Source: CAD feature listing. Evaluate the final solid. Frame: model axes, mm. Give positions to 0.01 mm unless a question says otherwise; leave off trailing zeros. Order: outer loops, then holes, each group sorted by start corner. A loop starts at its lowest first (then second) coordinate and runs counter-clockwise, first axis right, second up. Notation, with made-up numbers: M 16,-20 L 25,-20 A15 cw 25,-12 Z; hole C 55,68.25 d8. An arc over 180 degrees is marked long. Use CSV: the item, a comma, the result in double quotes. Start each with the question number.
1. Line query: line 1 along Y through (x, z) = (-40, 2.2); line 2 along Y through (x, z) = (0, 1.25). Output: solid intervals per line, ascending. Write a range as [from, to].
2. Section query C-C, the plane z = 2.6. Return the cut outline in (x, y) (1 decimal).
3. Section query D-D, the plane y = -35. Return the cut outline in (x, z) (3 decimals).
4. Section query A-A, the plane y = 0. Return the cut outline in (x, z) (1 decimal), plus the area to 4 significant figures.
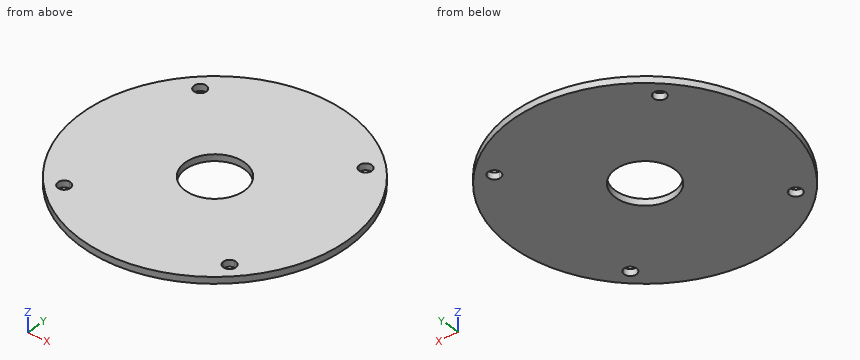
from build123d import *

# Parameters (mm, degrees)
F0_R     = 64.2875
F0_R_2   = 14.2875
F1_DEPTH = 3.175
F3_DEPTH = 25


with BuildPart() as f1:
    # F0 (on Top) → F1 (new body)
    with BuildSketch(Plane.XY):
        Circle(F0_R)
        Circle(F0_R_2, mode=Mode.SUBTRACT)
    extrude(amount=F1_DEPTH)

    # F2 (on face) → F3 (cut)
    with BuildSketch(Plane.XY.offset(3.175)):
        with BuildLine():
            ThreePointArc((-40, 37), (-37.87868, 37.87868), (-37, 40))
            Line((-37, 40), (-40, 40))
            Line((-40, 40), (-40, 37))
        make_face()
        with BuildLine():
            Line((-40, 40), (-37, 40))
            ThreePointArc((-37, 40), (-42.12132, 42.12132), (-40, 37))
            Line((-40, 37), (-40, 40))
        make_face()
        with BuildLine():
            Line((40, 40), (37, 40))
            ThreePointArc((37, 40), (37.87868, 37.87868), (40, 37))
            Line((40, 37), (40, 40))
        make_face()
        with BuildLine():
            ThreePointArc((43, 40), (40, 43), (37, 40))
            Line((37, 40), (40, 40))
            Line((40, 40), (40, 37))
            ThreePointArc((40, 37), (42.12132, 37.87868), (43, 40))
        make_face()
        with BuildLine():
            ThreePointArc((43, -40), (42.12132, -37.87868), (40, -37))
            Line((40, -37), (40, -40))
            Line((40, -40), (37, -40))
            ThreePointArc((37, -40), (40, -43), (43, -40))
        make_face()
        with BuildLine():
            Line((40, -40), (40, -37))
            ThreePointArc((40, -37), (37.87868, -37.87868), (37, -40))
            Line((37, -40), (40, -40))
        make_face()
        with BuildLine():
            Line((-40, -40), (-40, -37))
            ThreePointArc((-40, -37), (-42.12132, -42.12132), (-37, -40))
            Line((-37, -40), (-40, -40))
        make_face()
        with BuildLine():
            ThreePointArc((-37, -40), (-37.87868, -37.87868), (-40, -37))
            Line((-40, -37), (-40, -40))
            Line((-40, -40), (-37, -40))
        make_face()
    extrude(amount=-F3_DEPTH, mode=Mode.SUBTRACT)


solid = f1.part
Result set:
1,line 1,"[-50.33, -43], [-37, 37], [43, 50.33]"
1,line 2,"[-64.29, -14.29], [14.29, 64.29]"
2,outline,"C 0,0 d128.6; hole M -40,-37 A3 ccw long -37,-40 A3 ccw Z; hole M -40,37 A3 ccw -37,40 A3 ccw long Z; hole C 0,0 d28.6; hole M 37,-40 A3 ccw 43,-40 A3 ccw 40,-37 A3 ccw Z; hole M 37,40 A3 ccw 40,37 A3 ccw 43,40 A3 ccw Z"
3,outline,"M -53.925,0 L 53.925,0 L 53.925,3.175 L -53.925,3.175 Z"
4,outline,"M -64.3,0 L -14.3,0 L -14.3,3.2 L -64.3,3.2 Z; M 14.3,0 L 64.3,0 L 64.3,3.2 L 14.3,3.2 Z"
4,area,"317.5 mm2"
